Work out the finished part from the listing and answer in its coordinate system (mm). Give positions to 0.01 mm unless a question says otherwise; leave off trailing zeros. Order: outer loops, then holes, each group sorted by start corner. A loop starts at its lowest first (then second) coordinate and runs counter-clockwise, first axis right, second up. Notation, with made-up numbers: (34.5, -13) - (90.5, -13) arc R20 cw to (90.5, 15) - close; hole circle Ø3 at (54, 26). An arc over 180 degrees is marked (long way). Write each question's results on one line, items separated by ' | '.
from build123d import *

# Parameters (mm, degrees)
SKETCH_1_W          = 45
SKETCH_1_H          = 45
SKETCH_1_R          = 1.6
EXTRUDE_1_DEPTH     = 4
EXTRUDE_2_DEPTH     = 4
SKETCH_3_R          = 1.6
CUT_EXTRUDE_1_DEPTH = 4
FILLET_1_R          = 5
SKETCH_4_R          = 1.6
CUT_EXTRUDE_2_DEPTH = 4
SKETCH_5_R          = 12.744189695
SKETCH_5_R_2        = 10
CUT_EXTRUDE_3_DEPTH = 10
FILLET_2_R          = 5
FILLET_3_R          = 5


with BuildPart() as part:
    # 草图1 → 凸台-拉伸1 (new body)
    with BuildSketch(Plane.XY):
        Rectangle(SKETCH_1_W, SKETCH_1_H)
        with Locations((19, 0)):
            Circle(SKETCH_1_R, mode=Mode.SUBTRACT)
        with Locations(Location((-19, 0, 0), (0, 0, 180))):
            Circle(SKETCH_1_R, mode=Mode.SUBTRACT)
    extrude(amount=EXTRUDE_1_DEPTH)

    # 草图2 → 凸台-拉伸2 (add)
    with BuildSketch(Plane.XY.offset(4)):
        Polygon((52.5, 15), (22.5, 22.5), (22.5, 0), (52.5, 0), align=None)
        Polygon((52.5, 0), (22.5, 0), (22.5, -22.5), (52.5, -15), align=None)
    extrude(amount=-EXTRUDE_2_DEPTH)

    # 草图3 → 切除-拉伸1 (cut)
    with BuildSketch(Plane.XY.offset(4)):
        with Locations((27.5, 13)):
            Circle(SKETCH_3_R)
        with Locations((47.5, 13)):
            Circle(SKETCH_3_R)
        with Locations(Location((47.5, -13, 0), (0, 0, 180))):
            Circle(SKETCH_3_R)
        with Locations(Location((27.5, -13, 0), (0, 0, 180))):
            Circle(SKETCH_3_R)
    extrude(amount=-CUT_EXTRUDE_1_DEPTH, mode=Mode.SUBTRACT)

    # 圆角1
    fillet_1_edges = [part.edges().sort_by_distance(p)[0] for p in [
        (52.5, 15, 2),
        (52.5, -15, 2),
        (22.5, 22.5, 2),
    ]]
    fillet(fillet_1_edges, radius=FILLET_1_R)

    # 草图4 → 切除-拉伸2 (cut)
    with BuildSketch(Plane.XY.offset(4)):
        with Locations((0, 19)):
            Circle(SKETCH_4_R)
        with Locations(Location((0, -19, 0), (0, 0, 180))):
            Circle(SKETCH_4_R)
    extrude(amount=-CUT_EXTRUDE_2_DEPTH, mode=Mode.SUBTRACT)

    # 草图5 → 切除-拉伸3 (cut)
    with BuildSketch(Plane.XY.offset(4)):
        Circle(SKETCH_5_R)
        with Locations((37.5, 0)):
            Circle(SKETCH_5_R_2)
    extrude(amount=-CUT_EXTRUDE_3_DEPTH, mode=Mode.SUBTRACT)

    # 圆角2
    fillet_2_edges = [part.edges().sort_by_distance(p)[0] for p in [
        (-22.5, -22.5, 2),
        (-22.5, 22.5, 2),
    ]]
    fillet(fillet_2_edges, radius=FILLET_2_R)

    # 圆角3
    fillet_3_edges = [part.edges().sort_by_distance(p)[0] for p in [
        (22.5, -22.5, 2),
    ]]
    fillet(fillet_3_edges, radius=FILLET_3_R)


solid = part.part
1. A cutting plane is placed at A-A, the plane x = 19. Write down the section's boundary in (y, z), then the cut area to 3 significant figures.
Answer list:
outline: (-22.5, 0) - (-1.6, 0) - (-1.6, 4) - (-22.5, 4) - close; (1.6, 0) - (22.5, 0) - (22.5, 4) - (1.6, 4) - close | area: 167 mm^2
2. Determine the mould class of faces 1 (the face through (-22.5, 0, 2)), 2 (the face through (51.41, 14.21, 1.97)), 3 (the face through (-10.113, -7.755, 2.028)) for opening direction Y: +Y half, -Y half, draft (parallel to the pull), parting line (faces both ways), or undercut.
Answer list:
face 1: draft | face 2: +Y half | face 3: undercut
3. A cutting plane is placed at B-B, the plane y = 0. Write down the section's boundary in (x, z), then the cut area to 3 significant figures.
Answer list:
outline: (-22.5, 0) - (-20.6, 0) - (-20.6, 4) - (-22.5, 4) - close; (-17.4, 0) - (-12.74, 0) - (-12.74, 4) - (-17.4, 4) - close; (12.74, 0) - (17.4, 0) - (17.4, 4) - (12.74, 4) - close; (20.6, 0) - (27.5, 0) - (27.5, 4) - (20.6, 4) - close; (47.5, 0) - (52.5, 0) - (52.5, 4) - (47.5, 4) - close | area: 92.4 mm^2
4. A cutting plane is placed at D-D, the plane z = 1.25. State how many separate pieces and enclosed holes the cut face has, then the cut area to 3 significant figures.
Answer list:
separate pieces: 1 | enclosed holes: 10 | area: 2,240 mm^2
5. A cutting plane is placed at C-C, the plane x = 0. Write down the section's boundary in (y, z), then the cut area to 3 significant figures.
Answer list:
outline: (-22.5, 0) - (-20.6, 0) - (-20.6, 4) - (-22.5, 4) - close; (-17.4, 0) - (-12.74, 0) - (-12.74, 4) - (-17.4, 4) - close; (12.74, 0) - (17.4, 0) - (17.4, 4) - (12.74, 4) - close; (20.6, 0) - (22.5, 0) - (22.5, 4) - (20.6, 4) - close | area: 52.4 mm^2
6. Straight lines are drawn through the part: line 1 (Y direction, x = 0, z = 2.7); line 2 (X direction, y = -13, z = 0.8); line 3 (Y direction, x = 48, z = 3.1) (3 decimals). For each, find the intervals that lie inside material, in ascending order. Write a range as [from, to].
Answer list:
line 1: [-22.5, -20.6], [-17.4, -12.74], [12.74, 17.4], [20.6, 22.5] | line 2: [-22.5, 25.9], [29.1, 45.9], [49.1, 52.12] | line 3: [-16.125, -14.52], [-11.48, 11.48], [14.52, 16.125]
7. Given P1, Ø1, axis at y = -12, z = 0.5, coming from the +X side; P2, Ø4, axis at x = 0, y = 19, coming from the -Z side; P3, Ø1.5, axis at x = 39, z = 3.5, coming from the +Y side, each flat-ended and moving along its own axis, determine where each tip first touches the part or whether it passes through.
Answer list:
P1: x = 52.48 | P2: z = 0 | P3: y = 18.56
